from build123d import *

# Parameters (mm, degrees)
DODANIE_WYCI_GNI_CIE1_DEPTH      = 20
DODANIE_WYCI_GNI_CIE1_DEPTH_BACK = 20
SZKIC1_R                         = 7
SZKIC1_R_2                       = 4
DODANIE_WYCI_GNI_CIE2_DEPTH      = 10
DODANIE_WYCI_GNI_CIE2_DEPTH_BACK = 10
SZKIC2_R                         = 4
DODANIE_WYCI_GNI_CIE4_START      = -7
SZKIC3_W                         = 14
SZKIC3_H                         = 14
DODANIE_WYCI_GNI_CIE4_DEPTH      = 17
SZKIC9_R                         = 7
DODANIE_WYCI_GNI_CIE6_DEPTH      = 20
SZKIC4_R                         = 4
WYTNIJ_WYCI_GNI_CIE1_DEPTH       = 10
DODANIE_WYCI_GNI_CIE7_REACH      = 39.401
DODANIE_WYCI_GNI_CIE8_START      = -7
DODANIE_WYCI_GNI_CIE8_DEPTH      = 14
SZKIC11_R                        = 4
WYTNIJ_WYCI_GNI_CIE2_DEPTH       = 10
SZKIC12_R                        = 4
WYTNIJ_WYCI_GNI_CIE3_DEPTH       = 40.84971769
ZAOKR_GLENIE1_R                  = 2
WYTNIJ_WYCI_GNI_CIE4_DEPTH       = 1


with BuildPart() as part:
    # Szkic1 → Dodanie-wyciągnięcie1 (new, two sides: drawn at the far end of the back side and taken through both)
    with BuildSketch(Plane.XY.offset(-DODANIE_WYCI_GNI_CIE1_DEPTH_BACK)):
        Circle(SZKIC1_R)
        Circle(SZKIC1_R_2, mode=Mode.SUBTRACT)
    extrude(amount=DODANIE_WYCI_GNI_CIE1_DEPTH + DODANIE_WYCI_GNI_CIE1_DEPTH_BACK)

    # Szkic2 → Dodanie-wyciągnięcie2 (add, two sides: drawn at the far end of the back side and taken through both)
    with BuildSketch(Plane.XY.offset(-DODANIE_WYCI_GNI_CIE2_DEPTH_BACK)):
        Circle(SZKIC2_R)
    extrude(amount=DODANIE_WYCI_GNI_CIE2_DEPTH + DODANIE_WYCI_GNI_CIE2_DEPTH_BACK)

    # Szkic3 → Dodanie-wyciągnięcie4 (add)
    with BuildSketch(Plane(origin=(4.949747468, 4.949747468, 0), x_dir=(0, 0, 1), z_dir=(0.7071067811865438, 0.7071067811865512, 0)).offset(DODANIE_WYCI_GNI_CIE4_START)):
        Rectangle(SZKIC3_W, SZKIC3_H)
    extrude(amount=DODANIE_WYCI_GNI_CIE4_DEPTH)

    # Szkic9 → Dodanie-wyciągnięcie6 (add)
    with BuildSketch(Plane(origin=(0, 0, 0), x_dir=(0, 0, -1), z_dir=(1, 0, 0))):
        Circle(SZKIC9_R)
    extrude(amount=DODANIE_WYCI_GNI_CIE6_DEPTH)

    # Szkic4 → Wytnij-wyciągnięcie1 (cut)
    with BuildSketch(Plane(origin=(12.02081528, 12.02081528, 0), x_dir=(0, 0, -1), z_dir=(0.7071067811865438, 0.7071067811865513, 0))):
        with Locations(Location((0, 0, 0), (0, 0, 90))):
            Circle(SZKIC4_R)
    extrude(amount=-WYTNIJ_WYCI_GNI_CIE1_DEPTH, mode=Mode.SUBTRACT)

    # Szkic10 → Dodanie-wyciągnięcie7 (add, up to next)
    with BuildSketch(Plane(origin=(0, -7.5, 0), x_dir=(1, 0, 0), z_dir=(0, 1, 0)), mode=Mode.PRIVATE) as dodanie_wyci_gni_cie7_sk1:
        Polygon((-7, 20), (-7, -20), (7, -20), (7, -7), (20, -7), (20, 7), (7, 7), (7, 20), align=None)
    dodanie_wyci_gni_cie7_tool1 = extrude(dodanie_wyci_gni_cie7_sk1.sketch, amount=DODANIE_WYCI_GNI_CIE7_REACH, mode=Mode.PRIVATE) - part.part
    add(dodanie_wyci_gni_cie7_tool1.solids().sort_by_distance((3.311321, -7.5, 0))[0])

    # Dodanie-wyciągnięcie8: read off the stored shape, not the designer's step
    # Dodanie-wyciągnięcie8 outline → Dodanie-wyciągnięcie8 (add)
    with BuildSketch(Plane.XY.offset(DODANIE_WYCI_GNI_CIE8_START)):
        Polygon((16.970562748, -2), (16.970562748, 7.071067812), (9.899494937, 0), (8, -1.899494937), (8, -2), align=None)
    extrude(amount=DODANIE_WYCI_GNI_CIE8_DEPTH)

    # Szkic11 → Wytnij-wyciągnięcie2 (cut)
    with BuildSketch(Plane(origin=(20, 0, 0), x_dir=(0, 0, -1), z_dir=(1, 0, 0))):
        Circle(SZKIC11_R)
    extrude(amount=-WYTNIJ_WYCI_GNI_CIE2_DEPTH, mode=Mode.SUBTRACT)

    # Szkic12 → Wytnij-wyciągnięcie3 (cut, through all)
    with BuildSketch(Plane.XY.offset(10)):
        Circle(SZKIC12_R)
    extrude(amount=-WYTNIJ_WYCI_GNI_CIE3_DEPTH, mode=Mode.SUBTRACT)

    # Zaokrąglenie1
    zaokr_glenie1_edges = [part.edges().sort_by_distance(p)[0] for p in [
        (7.071067812, 16.970562748, 0),
    ]]
    fillet(zaokr_glenie1_edges, radius=ZAOKR_GLENIE1_R)

    # Szkic14 → Wytnij-wyciągnięcie4 (cut, along a direction that is not the sketch's normal)
    with BuildSketch(Plane(origin=(-4.949747468, 4.949747468, 0), x_dir=(0, 0, 1), z_dir=(-0.7071067811865513, 0.7071067811865438, 0))):
        Polygon((-2.075961538, 12.525), (2.564423077, 12.525), (2.564423077, 10.815384615), (-0.366346154, 10.815384615), (-0.366346154, 8.983653846), (2.564423077, 8.983653846), (2.564423077, 7.274038462), (-0.366346154, 7.274038462), (-0.366346154, 3), (-2.075961538, 3), align=None)
    extrude(amount=-WYTNIJ_WYCI_GNI_CIE4_DEPTH, dir=(0, 1, 0), mode=Mode.SUBTRACT)


solid = part.part
Read the model definition and answer for the solid it produces. Units are mm, in the model's axes. A direction names the side the tool comes from. Round coordinates to 2 decimals unless told otherwise and drop trailing zeros. Order: outer loops, then holes, each group sorted by start corner. A loop starts at its lowest first (then second) coordinate and runs counter-clockwise, first axis right, second up.
1) Flat-ended cylindrical pins translate along their axes: pin 1 (3 mm diameter, centred on y = -1, z = -16, fed in from +X); pin 2 (5 mm diameter, centred on y = 10.5, z = -6, fed in from -X); pin 3 (0.5 mm diameter, centred on y = 12, z = 0.5, fed in from +X). Find the tip coordinate at first contact, or state that the pin passes through.
2) Straight lines are drawn through the part: L1, parallel to Y at x = -3.5, z = 2.5; L2, parallel to X at y = -6.25, z = -13.5; L3, parallel to X at y = -2, z = 1. For each, find the intervals that lie inside material, in ascending order.
3) The part is cut by section C-C on y = -4.5. Write down the section's boundary in (x, z).
4) The mould has two halves that part along Z. Classify faces 4 (the face through (-0.9, 9, -0.1)), 5 (the face through (-1.3, 8.1, -0.366)): released by +Z, released by -Z, zero draft, split by the parting line, or undercut.
5) The part is cut by section A-A on x = -0.25. Write down the section's boundary in (y, z), plus the area to 3 significant figures.
6) For faces 1 (the face through (0.8, 10.2, 2.564)), 2 (the face through (5, 4.9, 0.1)), 3 (the face through (3.907, 13, 0)), determine the directions among +Z, -Z, +X, -X, +Y, -Y from which every point of the face is accessible in a straight line to the end or side of a thin tool.
7) The part is cut by section B-B on z = 13. Write down the section's boundary in (x, y).
Resolved:
1. pin 1: stops at x = 7
1. pin 2: stops at x = -1.9
1. pin 3: stops at x = 6.64
2. L1: y = -7.5 to -1.94, 1.94 to 6.4
2. L2: x = -7 to 7
2. L3: x = -7 to -3.46, 3.46 to 10
3. outline: (-7, -20) - (7, -20) - (7, -7) - (20, -7) - (20, 7) - (7, 7) - (7, 20) - (-7, 20) - close
4. face 4: zero draft
4. face 5: undercut
5. outline: (-7.5, -20) - (-3.99, -20) - (-3.99, 20) - (-7.5, 20) - close; (3.99, -20) - (7, -20) - (7, -7) - (9.65, -7) - (9.65, -2.08) - (8.65, -2.08) - (8.65, -0.37) - (9.65, -0.37) - (9.65, 7) - (7, 7) - (7, 20) - (3.99, 20) - close
5. area: 296 mm2
6. face 1: +Y
6. face 2: none
6. face 3: -X, +Y
7. outline: (-7, -7.5) - (7, -7.5) - (7, 0) arc R7 ccw to (-7, 0) - close; hole circle Ø8 at (0, 0)
